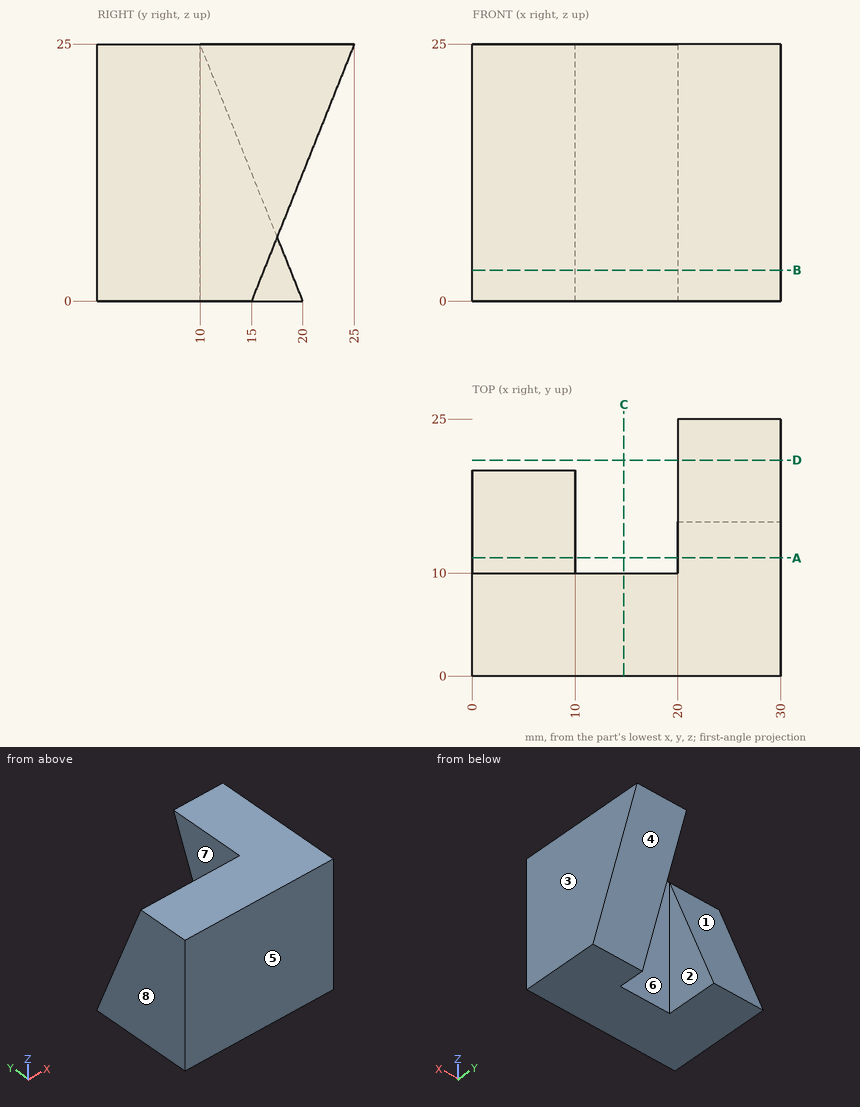
Answer from the drawing. Dimensions are ordinates in mm from the lowest x, y and z of the part. A direction names the side the tool comes from. Coordinates: 2 decimals unless noted, no trailing zeros. Loops run counter-clockwise (first coordinate to the right, second up) from the corner with the lowest first, then second, coordinate; pieces in that order, holes last.
1) Consider probe 1 along X at (y, z) = (10.75, 1.75); probe 2 along X at (y, z) = (20.5, 21); probe 3 along Y at (x, z) = (16.5, 15.75). Determine where each line is inside the solid, lowest interval first.
Results:
probe 1: x = 0 to 10, 20 to 30
probe 2: x = 20 to 30
probe 3: y = 0 to 10
2) For a pull along X with two mould halves and no side action, classify the marked faces 5, 6, 7 and 8 as +X half, -X half, draft (parallel to the pull), parting line (faces both ways), or undercut.
Results:
face 5: draft
face 6: undercut
face 7: undercut
face 8: -X half
3) For the marked faces 1, 2, 3 and 4, determine the directions among +Z, -Z, +X, -X, +Y, -Y from which every point of the face is accessible in a straight line to the end or side of a thin tool.
Results:
face 1: +Z, -X, +Y
face 2: +Z, -Z, +Y
face 3: +Z, -Z, +X, +Y, -Y
face 4: -Z, +X, +Y
4) Section A-A (y = 11.5) is taken. Give the vertices of the cut face in (x, z), plus the area to 4 significant figures.
Results:
outline: (0, 0) - (10, 0) - (10, 21.25) - (0, 21.25) - close; (20, 0) - (30, 0) - (30, 25) - (20, 25) - close
area: 462.5 mm2
5) Section C-C (x = 14.75) is taken. Give the vertices of the cut face in (y, z).
Results:
outline: (0, 0) - (10, 0) - (10, 25) - (0, 25) - close
6) Flat-ended cylindrical pins translate along their axes: pin 1 (5 mm diameter, centred on x = 4.5, y = 14, fed in from +Z); pin 2 (4 mm diameter, centred on x = 4.5, z = 5, fed in from +Y). Find the tip coordinate at first contact, or state that the pin passes through.
Results:
pin 1: stops at z = 21.25
pin 2: stops at y = 18.8
7) Section B-B (z = 3) is taken. Give the vertices of the cut face in (x, y).
Results:
outline: (0, 0) - (30, 0) - (30, 16.2) - (20, 16.2) - (20, 10) - (10, 10) - (10, 18.8) - (0, 18.8) - close
8) Section D-D (y = 21) is taken. Give the vertices of the cut face in (x, z).
Results:
outline: (20, 15) - (30, 15) - (30, 25) - (20, 25) - close
